Here's how the part is built. I have some questions about the finished solid (model axes, mm). Face numbers are marked on the shaded views. A direction names the side the tool comes from. Coordinates: 2 decimals unless noted, no trailing zeros. Loops run counter-clockwise (first coordinate to the right, second up) from the corner with the lowest first, then second, coordinate; pieces in that order, holes last.
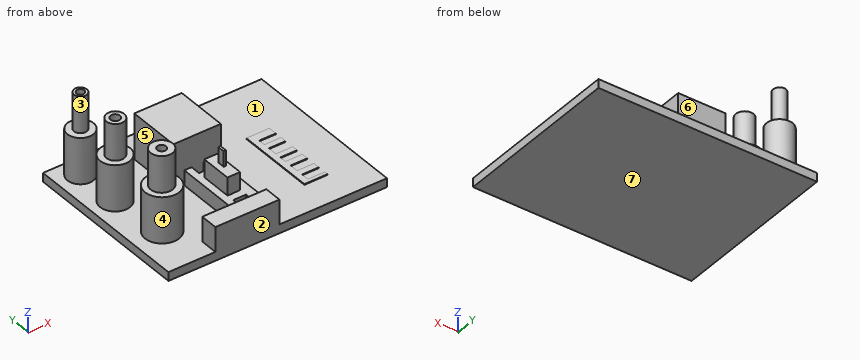
```python
from build123d import *

# Parameters (mm, degrees)
F0_W      = 360.8396798372
F0_H      = 281.035810709
F1_DEPTH  = 14.478
F2_R      = 21.5107094722
F2_R_2    = 24.7089721203
F2_R_3    = 28.2455541112
F3_DEPTH  = 75.692
F4_R      = 10.5555341184
F4_R_2    = 6.4147085914
F4_R_3    = 14.6610687467
F4_R_4    = 7.8515753599
F4_R_5    = 18.2872208754
F4_R_6    = 7.3119029403
F5_DEPTH  = 59.944
F6_W      = 78.4418359399
F6_H      = 87.4972045422
F7_DEPTH  = 74.93
F9_DEPTH  = 24.638
F10_W     = 20.9634182729
F10_H     = 51.7013933032
F11_DEPTH = 54.102
F12_W     = 3.7795142394
F12_H     = 12.0124146342
F13_DEPTH = 25.4
F14_W     = 105.7597789913
F14_H     = 29.3969660997
F15_DEPTH = 40.64
F17_DEPTH = 1.27


with BuildPart() as f1:
    # F0 (on Top) → F1 (new body)
    with BuildSketch(Plane.XY):
        with Locations((-14.175452292, -6.1578452587)):
            Rectangle(F0_W, F0_H)
    extrude(amount=-F1_DEPTH)

    # F2 (on face) → F3 (join)
    with BuildSketch(Plane.XY):
        with Locations((-157.2264283895, 101.2231707573)):
            Circle(F2_R)
        with Locations((-155.097797513, 26.4635402709)):
            Circle(F2_R_2)
        with Locations((-145.9769010544, -66.5491223335)):
            Circle(F2_R_3)
    extrude(amount=F3_DEPTH)

    # F4 (on face) → F5 (join)
    with BuildSketch(Plane.XY.offset(75.692)):
        with Locations((-157.2264283895, 101.2231707573)):
            Circle(F4_R)
        with Locations((-157.2264283895, 101.2231707573)):
            Circle(F4_R_2, mode=Mode.SUBTRACT)
        with Locations((-154.6684801579, 26.4845881611)):
            Circle(F4_R_3)
        with Locations((-154.6684801579, 26.4845881611)):
            Circle(F4_R_4, mode=Mode.SUBTRACT)
        with Locations((-146.3120281696, -65.9587830305)):
            Circle(F4_R_5)
        with Locations((-146.3120281696, -65.9587830305)):
            Circle(F4_R_6, mode=Mode.SUBTRACT)
    extrude(amount=F5_DEPTH)

    # F6 (on face) → F7 (join)
    with BuildSketch(Plane.XY):
        with Locations((-39.2209179699, 43.7486022711)):
            Rectangle(F6_W, F6_H)
    extrude(amount=F7_DEPTH)

    # F8 (on face) → F9 (join)
    with BuildSketch(Plane.XY):
        Polygon((-48.2832752168, 0), (-60.267470777, 0), (-60.267470777, -66.7334496975), (-60.267470777, -117.2787845135), (-48.2832752168, -117.2787845135), (-48.2832752168, -93.1336581707), (-48.2832752168, -80.6389690893), (-48.2832752168, -58.6393922567), (-48.2832752168, -43.9444051084), (-48.2832752168, -28.5100445064), (-48.2832752168, -16.6609026492), align=None)
        Polygon((-28.6240933259, -16.2599701732), (-48.2832752168, -16.6609026492), (-48.2832752168, -28.5100445064), (-28.3742633655, -28.5100445064), align=None)
        Polygon((-27.3198569439, -16.2333713694), (-28.6240933259, -16.2599701732), (-28.3742633655, -28.5100445064), align=None)
        Polygon((-28.9557017386, 0), (-28.6240933259, -16.2599701732), (-27.3198569439, -16.2333713694), (-28.3742633655, -28.5100445064), (-28.0799994067, -42.9388798786), (-27.3198569439, -58.211860977), (-27.7683332748, -58.2210072744), (-27.3198569439, -80.2114378095), (-26.5638995916, -93.1336581707), (-27.0563191308, -93.1336581707), (-26.5638995916, -117.2787845135), (-11.304622516, -117.2787845135), (-11.304622516, 0), align=None)
        Polygon((-48.2832752168, -80.6389690893), (-48.2832752168, -93.1336581707), (-27.0563191308, -93.1336581707), (-27.3198569439, -80.2114378095), align=None)
        Polygon((-27.3198569439, -80.2114378095), (-27.0563191308, -93.1336581707), (-26.5638995916, -93.1336581707), align=None)
    extrude(amount=F9_DEPTH)

    # F10 (on face) → F11 (join)
    with BuildSketch(Plane.XY):
        with Locations((-37.8015660804, -54.360741158)):
            Rectangle(F10_W, F10_H)
    extrude(amount=F11_DEPTH)

    # F12 (on face) → F13 (join)
    with BuildSketch(Plane.XY.offset(54.102)):
        with Locations((-35.9118089607, -51.5961125493)):
            Rectangle(F12_W, F12_H)
    extrude(amount=F13_DEPTH)

    # F14 (on face) → F15 (join)
    with BuildSketch(Plane.XY):
        with Locations((-64.1845120117, -131.9772675633)):
            Rectangle(F14_W, F14_H)
    extrude(amount=F15_DEPTH)

    # F16 (on face) → F17 (join)
    with BuildSketch(Plane.XY):
        Polygon((106.9932729006, 36.4078879356), (68.8668936491, 36.4078879356), (68.8668936491, -93.6395674944), (106.9932729006, -93.6395674944), (106.9932729006, -87.3722210526), (79.3124735355, -87.3722210526), (79.3124735355, -74.3152499199), (106.9932729006, -74.3152499199), (106.9932729006, -63.3473917842), (79.3124735355, -63.3473917842), (79.3124735355, -48.7235784531), (106.9932729006, -48.7235784531), (106.9932729006, -37.2334420681), (79.3124735355, -37.2334420681), (79.3124735355, -25.7433056831), (106.9932729006, -25.7433056831), (106.9932729006, -15.8200059086), (79.3124735355, -15.8200059086), (79.3124735355, 0), (106.9932729006, 0), (106.9932729006, 10.2939419448), (79.3124735355, 10.2939419448), (79.3124735355, 21.7840764672), (106.9932729006, 21.7840764672), align=None)
    extrude(amount=F17_DEPTH)


solid = f1.part
```
1. I want a section at C-C (z = 34.5). Please give me the cut outline in (x, y), then the cut area to 3 significant figures.
2. On a 3-axis mill with a long thin cutter (end or side, diameter ignored), from which of +Z, -Z, +X, -X, +Y, -Y can I reach the whole of each face in a straight line? I mean the marked faces 4, 5, 6 and 7. Say none if no direction works.
3. I want a section at A-A (x = 100.5). Please give me the cut outline in (y, z), then the cut area to 3 significant figures.
4. I want a section at D-D (z = 87). Please give me the cut outline in (x, y).
5. For pin 1 (5 mm diameter, centred on y = -88, z = 67.5, fed in from +X); pin 2 (0.6 mm diameter, centred on y = 29.5, z = 0.5, fed in from +X); pin 3 (4 mm diameter, centred on x = -134, z = 7, fed in from -Y), each with a flat end and sliding along its axis, tell me the tip position at first contact or that it passes through.
6. We'd pull the mould along X, two halves only. Please class the marked faces 1, 2 and 3: +X half, -X half, draft (parallel to the pull), parting line (faces both ways), or undercut.
7. I need wall thicknesses on line 1 along Y through (x, z) = (-145.5, 126); line 2 along Z through (x, y) = (-63, -117.5); line 3 along Z through (x, y) = (55, 65). Which ranges of each line are inside material? Lowest first, please.
8. I want a section at B-B (y = 63.5). Please give me the cut outline in (x, z), then the cut area to 3 significant figures.
Response values:
1. outline: circle Ø49.42 at (-155.1, 26.46); circle Ø43.02 at (-157.23, 101.22); circle Ø56.49 at (-145.98, -66.55); (-117.06, -146.68) - (-11.3, -146.68) - (-11.3, -117.28) - (-117.06, -117.28) - close; (-78.44, 0) - (0, 0) - (0, 87.5) - (-78.44, 87.5) - close; (-48.28, -80.21) - (-27.32, -80.21) - (-27.32, -28.51) - (-48.28, -28.51) - close
1. area: 16,900 mm2
2. face 4: +Z
2. face 5: +Z, +Y
2. face 6: +Z, +X, +Y
2. face 7: -Z, +X, -X, +Y, -Y
3. outline: (-146.68, -14.48) - (134.36, -14.48) - (134.36, 0) - (36.41, 0) - (36.41, 1.27) - (21.78, 1.27) - (21.78, 0) - (10.29, 0) - (10.29, 1.27) - (0, 1.27) - (0, 0) - (-15.82, 0) - (-15.82, 1.27) - (-25.74, 1.27) - (-25.74, 0) - (-37.23, 0) - (-37.23, 1.27) - (-48.72, 1.27) - (-48.72, 0) - (-63.35, 0) - (-63.35, 1.27) - (-74.32, 1.27) - (-74.32, 0) - (-87.37, 0) - (-87.37, 1.27) - (-93.64, 1.27) - (-93.64, 0) - (-146.68, 0) - close
3. area: 4,150 mm2
4. outline: circle Ø29.32 at (-154.67, 26.48); circle Ø21.11 at (-157.23, 101.22); circle Ø36.57 at (-146.31, -65.96); hole circle Ø12.83 at (-157.23, 101.22); hole circle Ø15.7 at (-154.67, 26.48); hole circle Ø14.62 at (-146.31, -65.96)
5. pin 1: stops at x = -125.03
5. pin 2: stops at x = 106.99
5. pin 3: stops at y = -92.97
6. face 1: undercut
6. face 2: draft
6. face 3: parting line
7. line 1: y = -84.23 to -73.23, -58.69 to -47.69, 15.04 to 37.93
7. line 2: z = -14.48 to 40.64
7. line 3: z = -14.48 to 0
8. outline: (-194.6, -14.48) - (166.24, -14.48) - (166.24, 0) - (0, 0) - (0, 74.93) - (-78.44, 74.93) - (-78.44, 0) - (-194.6, 0) - close
8. area: 11,100 mm2
